from build123d import *

# Parameters (mm, degrees)
GENERICCARDPCBDEFINITION_FILLET3_START   = -0.8
GENERICCARDPCBDEFINITION_FILLET3_OUTLI_R = 0.16
GENERICCARDPCBDEFINITION_FILLET3_DEPTH   = 1.6
SKETCH1_R                                = 1.1
CUT_EXTRUDE1_DEPTH                       = 10


# Read off the part's stored shape, not the designer's step: <GenericCardPCBDefinition>-<Fillet3>
with BuildPart() as part:
    # <GenericCardPCBDefinition>-<Fillet3> outli → <GenericCardPCBDefinition>-<Fillet3> (new body)
    with BuildSketch(Plane(origin=(0, 0, 0), x_dir=(1, 0, 0), z_dir=(0, 1, 0)).offset(GENERICCARDPCBDEFINITION_FILLET3_START)):
        with BuildLine():
            ThreePointArc((-41.232050808, -44.8), (-40.5, -44.067949192), (-39.5, -43.8))
            Line((-39.5, -43.8), (-38.267949192, -43.8))
            ThreePointArc((-38.267949192, -43.8), (-37.914395801, -43.653553391), (-37.767949192, -43.3))
            Line((-37.767949192, -43.3), (-37.767949192, -41.3))
            ThreePointArc((-37.767949192, -41.3), (-37.621502583, -40.946446609), (-37.267949192, -40.8))
            Line((-37.267949192, -40.8), (-35.59, -40.8))
            Line((-35.59, -40.8), (-35.59, -37.1))
            ThreePointArc((-35.59, -37.1), (-35.443553391, -36.746446609), (-35.09, -36.6))
            Line((-35.09, -36.6), (-32.91, -36.6))
            ThreePointArc((-32.91, -36.6), (-32.556446609, -36.746446609), (-32.41, -37.1))
            Line((-32.41, -37.1), (-32.41, -40.8))
            Line((-32.41, -40.8), (-29.59, -40.8))
            Line((-29.59, -40.8), (-29.59, -37.1))
            ThreePointArc((-29.59, -37.1), (-29.443553391, -36.746446609), (-29.09, -36.6))
            Line((-29.09, -36.6), (-26.91, -36.6))
            ThreePointArc((-26.91, -36.6), (-26.556446609, -36.746446609), (-26.41, -37.1))
            Line((-26.41, -37.1), (-26.41, -40.8))
            Line((-26.41, -40.8), (-23.59, -40.8))
            Line((-23.59, -40.8), (-23.59, -37.1))
            ThreePointArc((-23.59, -37.1), (-23.443553391, -36.746446609), (-23.09, -36.6))
            Line((-23.09, -36.6), (-20.91, -36.6))
            ThreePointArc((-20.91, -36.6), (-20.556446609, -36.746446609), (-20.41, -37.1))
            Line((-20.41, -37.1), (-20.41, -40.8))
            Line((-20.41, -40.8), (-18.732050808, -40.8))
            ThreePointArc((-18.732050808, -40.8), (-18.378497417, -40.946446609), (-18.232050808, -41.3))
            Line((-18.232050808, -41.3), (-18.232050808, -43.3))
            ThreePointArc((-18.232050808, -43.3), (-18.085604199, -43.653553391), (-17.732050808, -43.8))
            Line((-17.732050808, -43.8), (-16.5, -43.8))
            ThreePointArc((-16.5, -43.8), (-15.5, -44.067949192), (-14.767949192, -44.8))
            Line((-14.767949192, -44.8), (14.767949192, -44.8))
            ThreePointArc((14.767949192, -44.8), (16.5, -43.8), (18.232050808, -44.8))
            Line((18.232050808, -44.8), (37.767949192, -44.8))
            ThreePointArc((37.767949192, -44.8), (39.5, -43.8), (41.232050808, -44.8))
            Line((41.232050808, -44.8), (44.1, -44.8))
            Line((44.1, -44.8), (49.9, -39))
            Line((49.9, -39), (49.9, 40.7))
            ThreePointArc((49.9, 40.7), (49.753553391, 41.053553391), (49.4, 41.2))
            Line((49.4, 41.2), (47.65, 41.2))
            ThreePointArc((47.65, 41.2), (47.296446609, 41.346446609), (47.15, 41.7))
            Line((47.15, 41.7), (47.15, 46.4))
            ThreePointArc((47.15, 46.4), (47.003553391, 46.753553391), (46.65, 46.9))
            Line((46.65, 46.9), (34.9, 46.9))
            ThreePointArc((34.9, 46.9), (34.546446609, 47.046446609), (34.4, 47.4))
            Line((34.4, 47.4), (34.4, 49.3))
            ThreePointArc((34.4, 49.3), (34.253553391, 49.653553391), (33.9, 49.8))
            Line((33.9, 49.8), (-33.9, 49.8))
            ThreePointArc((-33.9, 49.8), (-34.253553391, 49.653553391), (-34.4, 49.3))
            Line((-34.4, 49.3), (-34.4, 47.4))
            ThreePointArc((-34.4, 47.4), (-34.546446609, 47.046446609), (-34.9, 46.9))
            Line((-34.9, 46.9), (-46.65, 46.9))
            ThreePointArc((-46.65, 46.9), (-47.003553391, 46.753553391), (-47.15, 46.4))
            Line((-47.15, 46.4), (-47.15, 41.7))
            ThreePointArc((-47.15, 41.7), (-47.296446609, 41.346446609), (-47.65, 41.2))
            Line((-47.65, 41.2), (-49.4, 41.2))
            ThreePointArc((-49.4, 41.2), (-49.753553391, 41.053553391), (-49.9, 40.7))
            Line((-49.9, 40.7), (-49.9, -39))
            Line((-49.9, -39), (-44.1, -44.8))
            Line((-44.1, -44.8), (-41.232050808, -44.8))
        make_face()
        with Locations((-35.59, -36.6)):
            Circle(GENERICCARDPCBDEFINITION_FILLET3_OUTLI_R, mode=Mode.SUBTRACT)
        with Locations((-32.41, -36.6)):
            Circle(GENERICCARDPCBDEFINITION_FILLET3_OUTLI_R, mode=Mode.SUBTRACT)
        with Locations((-29.59, -36.6)):
            Circle(GENERICCARDPCBDEFINITION_FILLET3_OUTLI_R, mode=Mode.SUBTRACT)
        with Locations((-26.41, -36.6)):
            Circle(GENERICCARDPCBDEFINITION_FILLET3_OUTLI_R, mode=Mode.SUBTRACT)
        with Locations((-23.59, -36.6)):
            Circle(GENERICCARDPCBDEFINITION_FILLET3_OUTLI_R, mode=Mode.SUBTRACT)
        with Locations((-20.41, -36.6)):
            Circle(GENERICCARDPCBDEFINITION_FILLET3_OUTLI_R, mode=Mode.SUBTRACT)
    extrude(amount=GENERICCARDPCBDEFINITION_FILLET3_DEPTH)

    # Sketch1 → Cut-Extrude1 (cut)
    with BuildSketch(Plane(origin=(0, 0.8, 0), x_dir=(1, 0, 0), z_dir=(0, 1, 0))):
        with Locations(Location((16.891859219, -16.911976124, 0), (0, 0, 270))):
            Circle(SKETCH1_R)
        with Locations(Location((16.891859219, 16.888023876, 0), (0, 0, 270))):
            Circle(SKETCH1_R)
        with Locations(Location((-16.908140781, -16.911976124, 0), (0, 0, 270))):
            Circle(SKETCH1_R)
        with Locations(Location((-16.908140781, 16.888023876, 0), (0, 0, 270))):
            Circle(SKETCH1_R)
        with BuildLine():
            Line((8.506216867, -8.611976124), (3, -8.611976124))
            Line((3, -8.611976124), (3, -9.511976124))
            ThreePointArc((3, -9.511976124), (-0.000900642, -12.511975988), (-2.999999459, -9.51017484))
            Line((-2.999999459, -9.51017484), (-2.997060521, -8.611976124))
            Line((-2.997060521, -8.611976124), (-8.493783133, -8.611976124))
            Line((-8.493783133, -8.611976124), (-8.493783133, 8.588023876))
            Line((-8.493783133, 8.588023876), (-3, 8.588023876))
            Line((-3, 8.588023876), (-3, 9.488023876))
            ThreePointArc((-3, 9.488023876), (0, 12.488023876), (3, 9.488023876))
            Line((3, 9.488023876), (3, 8.588023876))
            Line((3, 8.588023876), (8.506216867, 8.588023876))
            Line((8.506216867, 8.588023876), (8.506216867, -8.611976124))
        make_face()
    extrude(amount=-CUT_EXTRUDE1_DEPTH, mode=Mode.SUBTRACT)


solid = part.part
Geometry check sheet. Reference: the model listing, model coordinates, mm. A direction names the side the tool comes from. Coordinates: 2 decimals unless noted, no trailing zeros. Order: outer loops, then holes, each group sorted by start corner. A loop starts at its lowest first (then second) coordinate and runs counter-clockwise, first axis right, second up. Notation, with made-up numbers: (8.25, -26) - (48.25, -26) arc R7 ccw to (48.25, -14) - close; hole circle Ø6 at (11.25, 45). An arc over 180 degrees is marked (long way). Answer in a Markdown table with one row per item. Add a question column.
1) Material ranges on line 1 along X through (y, z) = (0.25, 39); line 2 along X through (y, z) = (0.35, -1); line 3 along X through (y, z) = (0.3, 17.5), recorded low to high. Write a range as [from, to].
2) Set-up check for faces 5 (the flat face through (-1, 0.8, -14)), 6 (the cylindrical face through (-0.066, 0.011, -12.487)): record each of +Z, -Z, +X, -X, +Y, -Y from which the full face is reachable in a straight line by a thin tool's end or side.
3) Release check for a two-part mould opening along X. For faces 1 (the flat face through (-1, -0.8, -14)), 2 (the cylindrical face through (15.82, 0.01, 16.67)), 3 (the flat face through (-47, 0, 41.9)), 4 (the flat face through (47, 0, 41.9)) record: +X half, -X half, draft (parallel to the pull), parting line (faces both ways), or undercut.
4) Gauge pin test, flat ends, axial feed: P1, Ø0.8, axis at x = -22, y = 0, coming from the +Z side; P2, Ø2, axis at x = 16.89, z = -16.89, coming from the +Y side; P3, Ø0.6, axis at x = -39, y = -0.5, coming from the +Z side. Record the tip position at first contact, or that the pin passes through.
5) Cross-section at B-B, the plane y = 0.4. State how many separate pieces and enclosed holes the cut face has, then the cut area to 3 significant figures.
6) Cross-section at A-A, the plane z = -2. Record the cut outline in (x, y).
Check result:
| question | item | result |
|---|---|---|
| 1 | line 1 | x = [-49.9, -35.59], [-32.41, -29.59], [-26.41, -23.59], [-20.41, 49.9] |
| 1 | line 2 | x = [-49.9, -8.49], [8.51, 49.9] |
| 1 | line 3 | x = [-49.9, -17.84], [-15.98, 15.96], [17.82, 49.9] |
| 2 | face 5 | +Z, -Z, +X, -X, +Y |
| 2 | face 6 | +Y, -Y |
| 3 | face 1 | draft |
| 3 | face 2 | undercut |
| 3 | face 3 | -X half |
| 3 | face 4 | +X half |
| 4 | P1 | stops at z = 36.6 |
| 4 | P2 | passes through |
| 4 | P3 | stops at z = 43.8 |
| 5 | separate pieces | 1 |
| 5 | enclosed holes | 11 |
| 5 | area | 8,810 mm² |
| 6 | outline | (-49.9, -0.8) - (-8.49, -0.8) - (-8.49, 0.8) - (-49.9, 0.8) - close; (8.51, -0.8) - (49.9, -0.8) - (49.9, 0.8) - (8.51, 0.8) - close |
